CAD build for the part. Positions are in the model's coordinates, mm. Face numbers are marked on the shaded views. A direction names the side the tool comes from. Round coordinates to 2 decimals unless told otherwise and drop trailing zeros. Loops run counter-clockwise (first coordinate to the right, second up) from the corner with the lowest first, then second, coordinate; pieces in that order, holes last. Notation, with made-up numbers: (21, 1.25) - (36, 1.25) arc R13 cw to (36, 21.25) - close; hole circle Ø7 at (61, 75.25). An arc over 180 degrees is marked (long way). One line per question, with ' | ' between items.
```python
from build123d import *

# Parameters (mm, degrees)
SKETCH1_W            = 200
SKETCH1_H            = 290
BOSS_EXTRUDE2_DEPTH  = 10
BOSS_EXTRUDE4_DEPTH  = 140
SKETCH5_W            = 20
SKETCH5_H            = 20
CUT_EXTRUDE1_DEPTH   = 10
SKETCH6_R            = 3.78
CUT_EXTRUDE2_DEPTH   = 10
SKETCH7_R            = 25
CUT_EXTRUDE3_DEPTH   = 10
SKETCH8_W            = 190
SKETCH8_H            = 280
CUT_EXTRUDE4_DEPTH   = 10
SKETCH9_W            = 211.457715155
SKETCH9_H            = 301.376650104
CUT_EXTRUDE5_DEPTH   = 5
SKETCH10_W           = 200
SKETCH10_H           = 5
BOSS_EXTRUDE7_DEPTH  = 15
SKETCH12_W           = 200
SKETCH12_H           = 5
BOSS_EXTRUDE8_DEPTH  = 15
SKETCH13_W           = 290
SKETCH13_H           = 5
BOSS_EXTRUDE14_DEPTH = 190
CUT_EXTRUDE6_DEPTH   = 300


with BuildPart() as part:
    # Sketch1 → Boss-Extrude2 (new body)
    with BuildSketch(Plane(origin=(0, 0, 0), x_dir=(1, 0, 0), z_dir=(0, 1, 0))):
        with Locations((3.938356164, -87.893835616)):
            Rectangle(SKETCH1_W, SKETCH1_H)
    extrude(amount=BOSS_EXTRUDE2_DEPTH)

    # Sketch2 → Boss-Extrude4 (add)
    with BuildSketch(Plane(origin=(0, 10, 0), x_dir=(1, 0, 0), z_dir=(0, 1, 0))):
        Polygon((-96.061643836, 57.106164384), (-96.061643836, -87.893835616), (-91.061643836, -87.893835616), (-91.061643836, 52.106164384), (3.938356164, 52.106164384), (3.938356164, 57.106164384), align=None)
        Polygon((103.938356164, 57.106164384), (3.938356164, 57.106164384), (3.938356164, 52.106164384), (98.938356164, 52.106164384), (98.938356164, -87.893835616), (103.938356164, -87.893835616), align=None)
        Polygon((3.938356164, -227.893835616), (3.938356164, -232.893835616), (103.938356164, -232.893835616), (103.938356164, -87.893835616), (98.938356164, -87.893835616), (98.938356164, -227.893835616), align=None)
        Polygon((-91.061643836, -87.893835616), (-96.061643836, -87.893835616), (-96.061643836, -232.893835616), (3.938356164, -232.893835616), (3.938356164, -227.893835616), (-91.061643836, -227.893835616), align=None)
    extrude(amount=BOSS_EXTRUDE4_DEPTH)

    # Sketch5 → Cut-Extrude1 (cut)
    with BuildSketch(Plane(origin=(103.938356164, 0, 0), x_dir=(0, 0, -1), z_dir=(1, 0, 0))):
        with Locations((-182.893835616, 112.5)):
            Rectangle(SKETCH5_W, SKETCH5_H)
        with Locations((-87.893835616, 112.5)):
            Rectangle(SKETCH5_W, SKETCH5_H)
        with Locations((7.106164384, 112.5)):
            Rectangle(SKETCH5_W, SKETCH5_H)
    extrude(amount=-CUT_EXTRUDE1_DEPTH, mode=Mode.SUBTRACT)

    # Sketch6 → Cut-Extrude2 (cut)
    with BuildSketch(Plane.ZY.offset(96.061643836)):
        with Locations((185.476335616, 112.5)):
            Circle(SKETCH6_R)
        with Locations((-9.688664384, 112.5)):
            Circle(SKETCH6_R)
        with Locations((185.476335616, 61.57)):
            Circle(SKETCH6_R)
        with Locations((-9.688664384, 61.57)):
            Circle(SKETCH6_R)
    extrude(amount=-CUT_EXTRUDE2_DEPTH, mode=Mode.SUBTRACT)

    # Sketch7 → Cut-Extrude3 (cut)
    with BuildSketch(Plane.XY.offset(232.893835616)):
        with Locations((63.938356164, 110)):
            Circle(SKETCH7_R)
    extrude(amount=-CUT_EXTRUDE3_DEPTH, mode=Mode.SUBTRACT)

    # Sketch8 → Cut-Extrude4 (cut)
    with BuildSketch(Plane(origin=(0, 10, 0), x_dir=(1, 0, 0), z_dir=(0, 1, 0))):
        with Locations((3.938356164, -87.893835616)):
            Rectangle(SKETCH8_W, SKETCH8_H)
    extrude(amount=-CUT_EXTRUDE4_DEPTH, mode=Mode.SUBTRACT)

    # Sketch9 → Cut-Extrude5 (cut)
    with BuildSketch(Plane.XZ):
        with Locations((3.40694666, 89.005470801)):
            Rectangle(SKETCH9_W, SKETCH9_H)
    extrude(amount=-CUT_EXTRUDE5_DEPTH, mode=Mode.SUBTRACT)

    # Sketch10 → Boss-Extrude7 (add)
    with BuildSketch(Plane(origin=(0, 0, 227.893835616), x_dir=(-1, 0, 0), z_dir=(0, 0, -1))):
        with Locations((-3.938356164, 147.5)):
            Rectangle(SKETCH10_W, SKETCH10_H)
    extrude(amount=BOSS_EXTRUDE7_DEPTH)

    # Sketch12 → Boss-Extrude8 (add)
    with BuildSketch(Plane.XY.offset(-52.106164384)):
        with Locations((3.938356164, 147.5)):
            Rectangle(SKETCH12_W, SKETCH12_H)
    extrude(amount=BOSS_EXTRUDE8_DEPTH)

    # Sketch13 → Boss-Extrude14 (add)
    with BuildSketch(Plane(origin=(-91.061643836, 0, 0), x_dir=(0, 0, -1), z_dir=(1, 0, 0))):
        with Locations((-87.893835616, 132.5)):
            Rectangle(SKETCH13_W, SKETCH13_H)
    extrude(amount=BOSS_EXTRUDE14_DEPTH)

    # Sketch17 → Cut-Extrude6 (cut)
    with BuildSketch(Plane.XY.offset(232.893835616)):
        Polygon((-16.061643836, 150), (-96.061643836, 150), (-16.061643836, 146.51), align=None)
        Polygon((103.938356164, 150), (-16.061643836, 150), (-16.061643836, 146.51), align=None)
    extrude(amount=-CUT_EXTRUDE6_DEPTH, mode=Mode.SUBTRACT)


solid = part.part
```
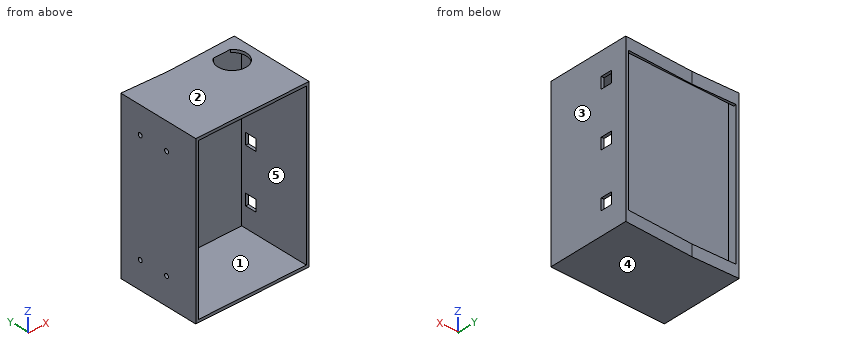
(1) Tool access for the marked faces 4 and 5: list every direction of +Z, -Z, +X, -X, +Y, -Y with a clear straight run to the whole face (end or side of a thin tool).
Results found:
face 4: -Z, +X, -X, +Y, -Y | face 5: -Y
(2) Cut at D-D, the plane x = 74.5. Write the cut outline in (y, z).
Results found:
outline: (5, -57.11) - (149.14, -57.11) - (149.14, -37.11) - (145, -37.11) - (145, -52.11) - (135, -52.11) - (135, 227.89) - (145, 227.89) - (145, 212.89) - (149.14, 212.89) - (149.14, 232.89) - (130, 232.89) - (130, -52.11) - (5, -52.11) - close; (5, 227.89) - (87.34, 227.89) - (87.34, 232.89) - (5, 232.89) - close
(3) Cut at B-B, the plane z = 197. Write the cut outline in (x, y), then the cut area to 3 significant figures.
Results found:
outline: (-96.06, 5) - (-91.06, 5) - (-91.06, 130) - (98.94, 130) - (98.94, 5) - (103.94, 5) - (103.94, 150) - (98.94, 149.85) - (98.94, 135) - (-91.06, 135) - (-91.06, 149.78) - (-96.06, 150) - close | area: 2,400 mm²
(4) Drop flat-ended pins along their axis: P1, Ø1.5, axis at x = 102.5, z = 184.5, coming from the +Y side; P2, Ø5, axis at x = -16.5, z = 65, coming from the +Y side; P3, Ø4.5, axis at y = 112.5, z = 185.48, coming from the +X side; P4, Ø4.5, axis at x = 12, z = 218, coming from the -Y side. Give the stop position or say it passes through.
Results found:
P1: stops at y = 149.98 | P2: stops at y = 135 | P3: passes through | P4: stops at y = 130
(5) Probe L1, parallel to Z at x = -92, y = 112; L2, parallel to Z at x = -82.5, y = 80; L3, parallel to X at y = 16.5, z = 102. List the from-to ranges inside material, lowest first.
Results found:
L1: z = -57.11 to -13.44, -5.94 to 181.73, 189.22 to 232.89 | L2: z = -57.11 to -52.11, 227.89 to 232.89 | L3: x = -96.06 to -91.06, 98.94 to 103.94
(6) Two-plate mould, pull along X, no slides. Class the marked faces 1, 2 and 3: released by +X, released by -X, zero draft, split by the parting line, or undercut.
Results found:
face 1: undercut | face 2: zero draft | face 3: released by +X
(7) Cut at C-C, the plane y = 61.57. Write the cut outline in (x, z), then the cut area to 3 significant figures.
Results found:
outline: (-96.06, -57.11) - (103.94, -57.11) - (103.94, 232.89) - (-96.06, 232.89) - (-96.06, 189.26) - (-91.06, 189.26) - (-91.06, 227.89) - (98.94, 227.89) - (98.94, -52.11) - (-91.06, -52.11) - (-91.06, -13.47) - (-96.06, -13.47) - close; (-96.06, -5.91) - (-91.06, -5.91) - (-91.06, 181.7) - (-96.06, 181.7) - close | area: 4,720 mm²
(8) Cut at A-A, the plane y = 47. Write the cut outline in (x, z), then the cut area to 3 significant figures.
Results found:
outline: (-96.06, -57.11) - (103.94, -57.11) - (103.94, 232.89) - (-96.06, 232.89) - close; hole (-91.06, -52.11) - (98.94, -52.11) - (98.94, 227.89) - (-91.06, 227.89) - close | area: 4,800 mm²
